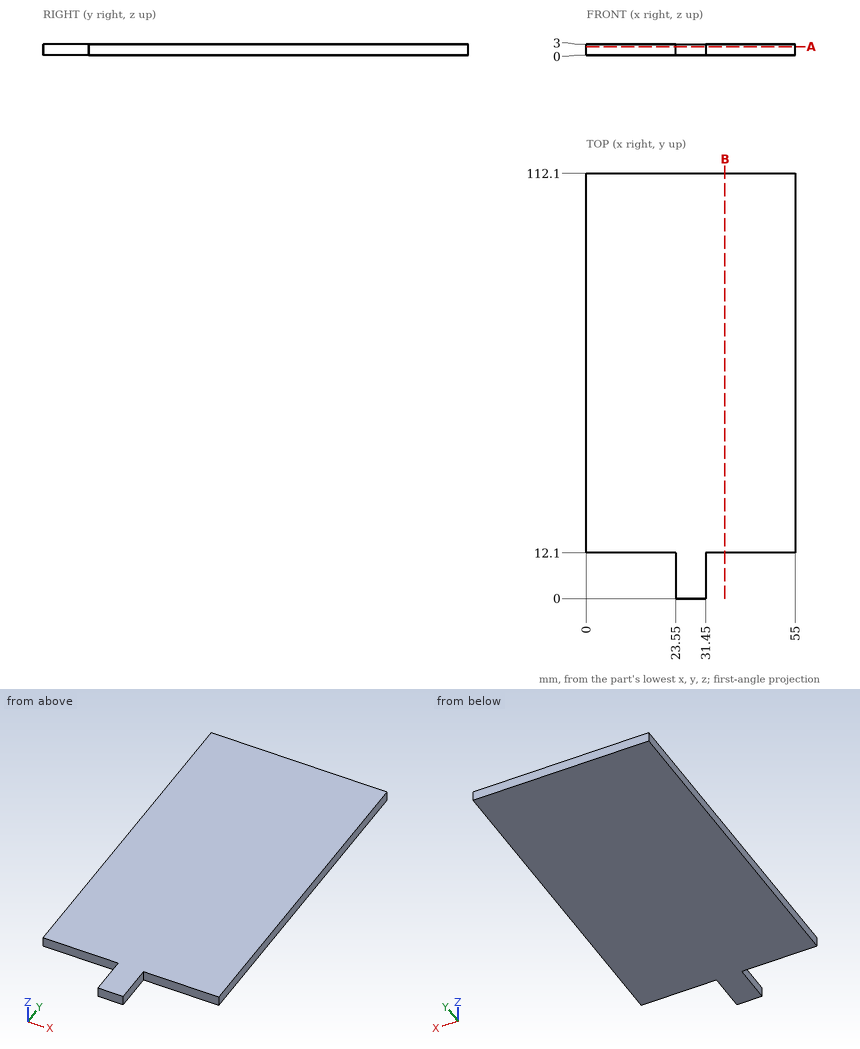
Job drawing, mm, ordinate dimensions from the low corner. One solid piece. Coordinates: 2 decimals unless noted, no trailing zeros. Order: outer loops, then holes, each group sorted by start corner. A loop starts at its lowest first (then second) coordinate and runs counter-clockwise, first axis right, second up. Notation, with made-up numbers: (-32, -26) - (27, -26) arc R21 ccw to (27, 11) - close; hole circle Ø6 at (28, -17). An arc over 180 degrees is marked (long way). Return JSON: item names as keys, results as strings. Group by question number.
1) Flat gauge pins, fed straight in: P1, Ø0.9, axis at y = 8, z = 2, coming from the +X side; P2, Ø0.9, axis at x = 44.5, z = 2, coming from the -Y side. Where does each tip first touch, or does it go through?
2) Saw through at B-B, the plane x = 36.5. Write the cut outline in (y, z).
3) Probe line 1 (Y direction, x = 52, z = 2.45); line 2 (X direction, y = 9, z = 2.5). List the from-to ranges inside material, lowest first. Write a range as from..to.
4) Saw through at A-A, the plane z = 2.3. Write the cut outline in (x, y), plus the area to 3 significant figures.
Values found:
{
 "1": {"P1": "stops at x = 31.45", "P2": "stops at y = 12.1"},
 "2": {"outline": "(12.1, 0) - (112.1, 0) - (112.1, 3) - (12.1, 3) - close"},
 "3": {"line 1": "y = 12.1..112.1", "line 2": "x = 23.55..31.45"},
 "4": {"outline": "(0, 12.1) - (23.55, 12.1) - (23.55, 0) - (31.45, 0) - (31.45, 12.1) - (55, 12.1) - (55, 112.1) - (0, 112.1) - close", "area": "5,600 mm²"}
}
